Check sheet for the modelled part. Datum: model origin and axes. Units: mm. Face numbers are marked on the shaded views. A direction names the side the tool comes from. Coordinates: 2 decimals unless noted, no trailing zeros. Loops run counter-clockwise (first coordinate to the right, second up) from the corner with the lowest first, then second, coordinate; pieces in that order, holes last.
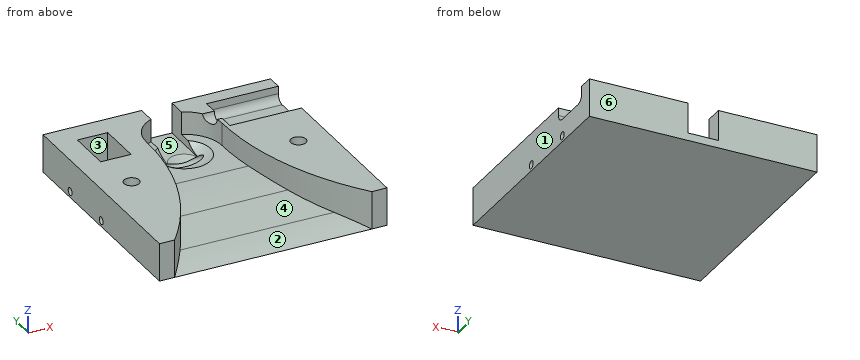
from build123d import *

# Parameters (mm, degrees)
F1_DEPTH  = 25
F3_DEPTH  = 150
F7_R      = 2.5
F8_DEPTH  = 150.001
F9_W      = 20
F9_H      = 30
F9_R      = 5
F9_H_2    = 35
F10_DEPTH = 20
F12_DEPTH = 47.3
F13_R     = 5
F14_DEPTH = 15.8


with BuildPart() as f1:
    # F0 (on Top) → F1 (new body)
    with BuildSketch(Plane.XY):
        with BuildLine():
            Line((75, 75), (-75, 75))
            Line((-75, 75), (-75, -75))
            Line((-75, -75), (-65, -75))
            ThreePointArc((-65, -75), (-35.2854373604, -20.8789783094), (-25, 40))
            ThreePointArc((-25, 40), (0, 65), (25, 40))
            ThreePointArc((25, 40), (35.2854373604, -20.8789783094), (65, -75))
            Line((65, -75), (75, -75))
            Line((75, -75), (75, 75))
        make_face()
    extrude(amount=F1_DEPTH)

    # F2 (on face) → F3 (join, through all)
    with BuildSketch(Plane(origin=(-75, 0, 0), x_dir=(0, -1, 0), z_dir=(-1, 0, 0))):
        with BuildLine():
            Line((-75, 10), (-75, 0))
            Line((-75, 0), (75, 0))
            ThreePointArc((75, 0), (64.7364457874, 2.863347323), (54.2264872704, 4.6183615505))
            Line((54.2264872704, 4.6183615505), (23.1799102031, 8.115113068))
            ThreePointArc((23.1799102031, 8.115113068), (6.4181072647, 9.5284076014), (-10.3965601359, 10))
            Line((-10.3965601359, 10), (-75, 10))
        make_face()
    extrude(amount=-F3_DEPTH)

    # F5 (on offset) → F6 (revolve, cut)
    with BuildSketch(Plane.XY.offset(28)):
        with BuildLine():
            Line((-25, 40), (25, 40))
            ThreePointArc((25, 40), (0, 65), (-25, 40))
        make_face()
    revolve(axis=Axis((0, 40, 28), (-1, 0, 0)), mode=Mode.SUBTRACT)

    # F7 (on face) → F8 (cut, through all)
    with BuildSketch(Plane.YZ.offset(75)):
        with Locations((40, 4)):
            Circle(F7_R)
        with Locations((0, 4)):
            Circle(F7_R)
    extrude(amount=-F8_DEPTH, mode=Mode.SUBTRACT)

    # F9 (on face) → F10 (cut)
    with BuildSketch(Plane.XY.offset(25)):
        with Locations((-50, 45)):
            Rectangle(F9_W, F9_H)
        with Locations((-55, 0)):
            Circle(F9_R)
        with Locations((55, 0)):
            Circle(F9_R)
        with Locations((0, 57.5)):
            Rectangle(F9_W, F9_H_2)
    extrude(amount=-F10_DEPTH, mode=Mode.SUBTRACT)

    # F11 (on face) → F12 (cut)
    with BuildSketch(Plane.YZ.offset(75)):
        with BuildLine():
            Line((65, 25), (35, 25))
            Line((35, 25), (35, 20))
            ThreePointArc((35, 20), (36.4644660941, 16.4644660941), (40, 15))
            Line((40, 15), (60, 15))
            ThreePointArc((60, 15), (63.5355339059, 16.4644660941), (65, 20))
            Line((65, 20), (65, 25))
        make_face()
    extrude(amount=-F12_DEPTH, mode=Mode.SUBTRACT)

    # F13 (on face) → F14 (cut)
    with BuildSketch(Plane.YZ.offset(27.7)):
        with Locations((50, 25)):
            Circle(F13_R)
    extrude(amount=-F14_DEPTH, mode=Mode.SUBTRACT)


solid = f1.part
(1) Draft check along Y on the marked faces 3, 4, 5 and 6. Enter one of: pulls with the +Y half, pulls with the -Y half, needs draft (parallel to the pull), parting line crosses it, or undercut.
(2) Section check C-C, the plane y = 16. Enter the section's corners in (x, z).
(3) Scan lines: line 1 along Y through (x, z) = (55, 16.5); line 2 along Y through (x, z) = (-55, 23.5); line 3 along X through (y, z) = (0, 17). Record each from-to range of solid material in increasing order.
(4) Section check A-A, the plane x = -63. Enter the section's corners in (y, z).
(5) Set-up check for the marked faces 1 and 2: record each of +Z, -Z, +X, -X, +Y, -Y from which the full face is reachable in a straight line by a thin tool's end or side.
(6) Section check D-D, the plane x = -46.5. Enter the section's corners in (y, z).
(7) Gauge pin test, flat ends, axial feed: P1, Ø12, axis at x = -26, y = -17.5, coming from the +Z side; P2, Ø6.5, axis at y = 0, z = 4, coming from the -X side; P3, Ø10, axis at x = 52, y = 53, coming from the +Z side; P4, Ø2.5, axis at x = 59, z = 23, coming from the -Y side. Record the tip position at first contact, or that the pin passes through.
(8) Section check B-B, the plane x = 57. Enter the section's corners in (y, z), plus the area to 3 significant figures.
Determined:
1. face 3: undercut
1. face 4: pulls with the -Y half
1. face 5: needs draft
1. face 6: pulls with the +Y half
2. outline: (-75, 0) - (75, 0) - (75, 25) - (26.56, 25) - (26.56, 10) - (-26.56, 10) - (-26.56, 25) - (-75, 25) - close
3. line 1: y = -61.09 to -5, 5 to 36.43, 63.57 to 75
3. line 2: y = -61.09 to -5, 5 to 30, 60 to 75
3. line 3: x = -75 to -60, -50 to -29.37, 29.37 to 50, 60 to 75
4. outline: (-75, 0) - (75, 0) - (75, 25) - (-72.43, 25) - (-72.43, 0.83) arc R100 ccw to start; hole circle Ø5 at (0, 4); hole circle Ø5 at (40, 4)
5. face 1: +Z, -Z, +X, +Y, -Y
5. face 2: +Z, -Y
6. outline: (-75, 0) - (75, 0) - (75, 25) - (60, 25) - (60, 5) - (42.29, 5) arc R2.5 cw (long way) to (37.71, 5) - (30, 5) - (30, 25) - (-46.64, 25) - (-46.64, 5.47) - (-54.23, 4.62) arc R100 ccw to start; hole circle Ø5 at (0, 4)
7. P1: stops at z = 9.2
7. P2: stops at x = -75
7. P3: stops at z = 15
7. P4: stops at y = -68.73
8. outline: (-75, 0) - (75, 0) - (75, 25) - (65, 25) - (65, 20) arc R5 cw to (60, 15) - (40, 15) arc R5 cw to (35, 20) - (35, 25) - (4.58, 25) - (4.58, 5) - (2.29, 5) arc R2.5 cw (long way) to (-2.29, 5) - (-4.58, 5) - (-4.58, 25) - (-64.1, 25) - (-64.1, 3) arc R100 ccw to start; hole circle Ø5 at (40, 4)
8. area: 2,990 mm2
